from build123d import *

# Parameters (mm, degrees)
F0_R     = 1
F1_DEPTH = 2
F2_R     = 1
F3_DEPTH = 9


# Not quite as in the source:
# - a feature of the source that left no trace in its solid (it failed there, or was rolled back) is left out


with BuildPart() as f1:
    # F0 (on Front) → F1 (new body)
    with BuildSketch(Plane.XZ):
        Polygon((-2, 1.1547005384), (-2, -1.1547005384), (0, -2.3094010768), (2, -1.1547005384), (2, 1.1547005384), (0, 2.3094010768), align=None)
        Circle(F0_R, mode=Mode.SUBTRACT)
        Circle(F0_R)
    extrude(amount=F1_DEPTH)

    # F2 (on face) → F3 (join)
    with BuildSketch(Plane(origin=(0, 0, 0), x_dir=(-1, 0, 0), z_dir=(0, 1, 0))):
        Circle(F2_R)
    extrude(amount=F3_DEPTH)


solid = f1.part
The listing builds one solid part. Answer for the finished solid, in the listing's coordinates (mm). A direction names the side the tool comes from. Round coordinates to 2 decimals unless told otherwise and drop trailing zeros. Loops run counter-clockwise (first coordinate to the right, second up) from the corner with the lowest first, then second, coordinate; pieces in that order, holes last. Notation, with made-up numbers: M 54,5 L 86,5 A31 ccw 86,29 Z; hole C 15,14 d6. An arc over 180 degrees is marked long. Write each question's results on one line, items separated by ' | '. Start each with the question number.
1) Straight lines are drawn through the part: probe 1 along Y at (x, z) = (0.3, -1.15); probe 2 along X at (y, z) = (-1, 1.6); probe 3 along Z at (x, y) = (0.45, 7). For each, find the intervals that lie inside material, in ascending order.
2) Each of these flat-tipped pins is pushed along its axis until it touches: pin 1 (1.5 mm diameter, centred on x = 1, y = 0.5, fed in from +Z); pin 2 (1 mm diameter, centred on x = -1, y = 2.5, fed in from +Z); pin 3 (1 mm diameter, centred on x = -0.5, y = 7, fed in from +Z). Where does it stop, or does it pass through?
3) Which of the six approach directions +Z, -Z, +X, -X, +Y, -Y give full straight-line access (tool end or side, diameter ignored) to faces 1 (the cylindrical face through (0, 4, -1)), 2 (the flat face through (0.99, -0.99, -1.74))?
4) Find section D-D on z = 1.55. Write down the section's boundary in (x, y), plus the area to 3 significant figures.
5) Find section C-C on y = 1.5. Write down the section's boundary in (x, z), plus the area to 3 significant figures.
6) Find section A-A on z = 0. Write down the section's boundary in (x, y), plus the area to 3 significant figures.
7) Find section B-B on x = 0.5. Write down the section's boundary in (y, z), plus the area to 3 significant figures.
Final values:
1) probe 1: -2 to 0 | probe 2: -1.23 to 1.23 | probe 3: -0.89 to 0.89
2) pin 1: z = 2.05 | pin 2: z = 0.87 | pin 3: z = 1
3) face 1: +Y | face 2: -Z, +X, +Y, -Y
4) outline: M -1.32,-2 L 1.32,-2 L 1.32,0 L -1.32,0 Z | area: 5.26 mm²
5) outline: C 0,0 d2 | area: 3.14 mm²
6) outline: M -2,-2 L 2,-2 L 2,0 L 1,0 L 1,9 L -1,9 L -1,0 L -2,0 Z | area: 26.0 mm²
7) outline: M -2,-2.02 L 0,-2.02 L 0,-0.87 L 9,-0.87 L 9,0.87 L 0,0.87 L 0,2.02 L -2,2.02 Z | area: 23.7 mm²
